```python
from build123d import *

# Parameters (mm, degrees)
SKETCH1_W           = 31
SKETCH1_H           = 80
BOSS_EXTRUDE1_DEPTH = 4
SKETCH2_W           = 24
SKETCH2_H           = 2.5
CUT_EXTRUDE1_DEPTH  = 3
BOSS_EXTRUDE2_DEPTH = 12
CUT_EXTRUDE3_DEPTH  = 7
SKETCH5_W           = 22.630422209
SKETCH5_H           = 4
BOSS_EXTRUDE3_DEPTH = 2
CHAMFER1_SIZE       = 2
CHAMFER2_SIZE       = 2
CHAMFER3_SIZE       = 2
CHAMFER4_SIZE       = 2
CHAMFER6_SIZE       = 1


with BuildPart() as part:
    # Sketch1 → Boss-Extrude1 (new body)
    with BuildSketch(Plane(origin=(0, 0, 0), x_dir=(1, 0, 0), z_dir=(0, 1, 0))):
        with Locations((-0.854779412, 28.517463235)):
            Rectangle(SKETCH1_W, SKETCH1_H)
    extrude(amount=BOSS_EXTRUDE1_DEPTH)

    # Sketch2 → Cut-Extrude1 (cut)
    with BuildSketch(Plane.XZ):
        with Locations((-0.854779412, 8.232536765)):
            Rectangle(SKETCH2_W, SKETCH2_H)
    extrude(amount=-CUT_EXTRUDE1_DEPTH, mode=Mode.SUBTRACT)

    # Sketch3 → Boss-Extrude2 (add)
    with BuildSketch(Plane.XZ):
        Polygon((-16.354779412, 6.982536765), (-12.354779412, 6.982536765), (-12.354779412, -64.517463235), (10.645220588, -64.517463235), (10.645220588, 6.982536765), (14.645220588, 6.982536765), (14.645220588, -68.517463235), (10.645220588, -68.517463235), (-12.354779412, -68.517463235), (-16.354779412, -68.517463235), align=None)
    extrude(amount=BOSS_EXTRUDE2_DEPTH)

    # Sketch4 → Cut-Extrude3 (cut)
    with BuildSketch(Plane.XZ.offset(12)):
        Polygon((-15.554779412, 6.982536765), (-13.154779412, 6.982536765), (-13.154779412, -65.317463235), (-12.154779412, -65.317463235), (-12.154779412, -67.717463235), (-13.154779412, -67.717463235), (-15.554779412, -67.717463235), align=None)
        Polygon((11.445220588, 6.982536765), (13.845220588, 6.982536765), (13.845220588, -67.717463235), (11.445220588, -67.717463235), (10.445220588, -67.717463235), (10.445220588, -65.317463235), (11.445220588, -65.317463235), align=None)
    extrude(amount=-CUT_EXTRUDE3_DEPTH, mode=Mode.SUBTRACT)

    # Sketch5 → Boss-Extrude3 (add)
    with BuildSketch(Plane.XZ.offset(12)):
        with Locations((-0.839568307, -66.517463235)):
            Rectangle(SKETCH5_W, SKETCH5_H)
    extrude(amount=BOSS_EXTRUDE3_DEPTH)

    # Chamfer1
    chamfer1_edges = [part.edges().sort_by_distance(p)[0] for p in [
        (-16.354779412, 2, 11.482536765),
        (14.645220588, 2, 11.482536765),
    ]]
    chamfer(chamfer1_edges, length=CHAMFER1_SIZE)

    # Chamfer2
    chamfer2_edges = [part.edges().sort_by_distance(p)[0] for p in [
        (-0.854779412, 4, 11.482536765),
    ]]
    chamfer(chamfer2_edges, length=CHAMFER2_SIZE)

    # Chamfer3
    chamfer3_edges = [part.edges().sort_by_distance(p)[0] for p in [
        (-16.354779412, 4, -29.517463235),
        (14.645220588, 4, -29.517463235),
    ]]
    chamfer(chamfer3_edges, length=CHAMFER3_SIZE)

    # Chamfer4
    chamfer4_edges = [part.edges().sort_by_distance(p)[0] for p in [
        (-0.854779412, 4, -68.517463235),
    ]]
    chamfer(chamfer4_edges, length=CHAMFER4_SIZE)

    # Chamfer6
    chamfer6_edges = [part.edges().sort_by_distance(p)[0] for p in [
        (14.645220588, -5, -68.517463235),
        (-16.354779412, -5, -68.517463235),
    ]]
    chamfer(chamfer6_edges, length=CHAMFER6_SIZE)


solid = part.part
```
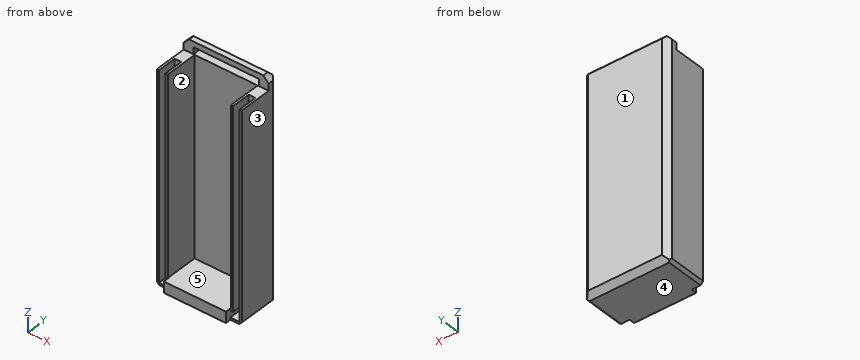
Work out the finished part from the listing and answer in its coordinate system (mm). Face numbers are marked on the shaded views. A direction names the side the tool comes from. Round coordinates to 2 decimals unless told otherwise and drop trailing zeros. Order: outer loops, then holes, each group sorted by start corner. A loop starts at its lowest first (then second) coordinate and runs counter-clockwise, first axis right, second up.
Q1. Given pin 1 Ø1.7 at (x, y) = (12.5, -8) entering from +Z; pin 2 Ø2 at (x, z) = (-8.5, 10) entering from -Y; pin 3 Ø2 at (x, z) = (-14.5, -26) entering from -Y, each flat-ended and moving along its own axis, determine where each tip first touches the part or whether it passes through.
Solution:
pin 1: stops at z = -67.72
pin 2: stops at y = 0
pin 3: stops at y = -5
Q2. The mould has two halves that part along X. Classify the marked faces 1, 2 and 3: pulls with the +X half, pulls with the -X half, needs draft (parallel to the pull), parting line crosses it, or undercut.
Solution:
face 1: needs draft
face 2: undercut
face 3: pulls with the +X half
Q3. A tool of negligible diameter and unlimited length cuts with its end or side. For the marked faces 4 and 5, from which of +Z, -Z, +X, -X, +Y, -Y can it reach the whole face along a straight path? Write none if from no direction.
Solution:
face 4: -Z, +X, -X, +Y, -Y
face 5: +Z, -Y
Q4. A cutting plane is placed at D-D, the plane y = -7. Determine the outline of the cut face in (x, z).
Solution:
outline: (-16.35, -67.52) - (-15.35, -68.52) - (13.65, -68.52) - (14.65, -67.52) - (14.65, 6.98) - (13.85, 6.98) - (13.85, -67.72) - (10.45, -67.72) - (10.45, -65.32) - (11.45, -65.32) - (11.45, 6.98) - (10.65, 6.98) - (10.65, -64.52) - (-12.35, -64.52) - (-12.35, 6.98) - (-13.15, 6.98) - (-13.15, -65.32) - (-12.15, -65.32) - (-12.15, -67.72) - (-15.55, -67.72) - (-15.55, 6.98) - (-16.35, 6.98) - close
Q5. Find the intervals of material crossed by line 1 along X through (y, z) = (-5.5, -32.5); line 2 along Z through (x, y) = (7.5, 0.5); line 3 along X through (y, z) = (2.5, -7), in increasing order.
Solution:
line 1: x = -16.35 to -15.55, -13.15 to -12.35, 10.65 to 11.45, 13.85 to 14.65
line 2: z = -68.52 to 6.98, 9.48 to 11.48
line 3: x = -15.85 to 14.15
Q6. A cutting plane is placed at C-C, the plane x = -5. Determine the outline of the cut face in (y, z).
Solution:
outline: (-14, -68.52) - (2, -68.52) - (4, -66.52) - (4, 9.48) - (2, 11.48) - (0, 11.48) - (0, 9.48) - (3, 9.48) - (3, 6.98) - (0, 6.98) - (0, -64.52) - (-14, -64.52) - close
Q7. A cutting plane is placed at B-B, the plane z = -49.5. Determine the outline of the cut face in (x, y).
Solution:
outline: (-16.35, -12) - (-15.55, -12) - (-15.55, -5) - (-13.15, -5) - (-13.15, -12) - (-12.35, -12) - (-12.35, 0) - (10.65, 0) - (10.65, -12) - (11.45, -12) - (11.45, -5) - (13.85, -5) - (13.85, -12) - (14.65, -12) - (14.65, 2) - (12.65, 4) - (-14.35, 4) - (-16.35, 2) - close
Q8. A cutting plane is placed at A-A, the plane y = 1.25. Determine the outline of the cut face in (x, z).
Solution:
outline: (-16.35, -67.52) - (-15.35, -68.52) - (13.65, -68.52) - (14.65, -67.52) - (14.65, 9.48) - (12.65, 11.48) - (-14.35, 11.48) - (-16.35, 9.48) - close; hole (-12.85, 6.98) - (11.15, 6.98) - (11.15, 9.48) - (-12.85, 9.48) - close
